from build123d import *

# Parameters (mm, degrees)
F0_W     = 90
F0_H     = 5
F1_DEPTH = 1
F0_W_2   = 5
F0_H_2   = 20
F2_DEPTH = 10
F3_W     = 90
F3_H     = 1
F4_DEPTH = 2
F5_SIZE  = 3
F6_SIZE  = 1
F7_SIZE  = 5


with BuildPart() as f1:
    # F0 (on Top) → F1 (new body)
    with BuildSketch(Plane.XY):
        with Locations((5, -7.5)):
            Rectangle(F0_W, F0_H)
    extrude(amount=F1_DEPTH)



with BuildPart() as f1b:
    # F0 (on Top) → F1, piece 2 (new body)
    with BuildSketch(Plane.XY):
        Polygon((50, 5), (50, 10), (-30, 10), (-40, 10), (-40, 5), align=None)
    extrude(amount=F1_DEPTH)


with BuildPart() as f1_1:
    add(f1.part)

    add(f1b.part)  # F2 merges F1b
    # F0 (on Top) → F2 (join)
    with BuildSketch(Plane.XY):
        Polygon((70, -10), (70, 10), (50, 10), (50, 5), (50, -5), (50, -10), align=None)
        Polygon((-45, 10), (-40, 10), (-40, 15), (-70, 15), (-70, 10), (-65, 10), align=None)
        Polygon((-40, 5), (-40, 10), (-45, 10), (-45, -10), (-40, -10), (-40, -5), align=None)
        with Locations((-67.5, 0)):
            Rectangle(F0_W_2, F0_H_2)
        Polygon((-40, -15), (-40, -10), (-45, -10), (-65, -10), (-70, -10), (-70, -15), align=None)
    extrude(amount=F2_DEPTH)

    # F3 (on face) → F4 (join)
    with BuildSketch(Plane.XY.offset(1)):
        with Locations((5, 5.5)):
            Rectangle(F3_W, F3_H)
        with Locations((5, -5.5)):
            Rectangle(F3_W, F3_H)
    extrude(amount=F4_DEPTH)

    # F5
    f5_edges = [f1_1.edges().sort_by_distance(p)[0] for p in [
        (70, -10, 5),
        (70, 10, 5),
        (50, -10, 5.5),
        (50, 10, 5.5),
    ]]
    chamfer(f5_edges, length=F5_SIZE)

    # F6
    f6_edges = [f1_1.edges().sort_by_distance(p)[0] for p in [
        (60, 10, 10),
        (51.5, 8.5, 10),
        (50, 0, 10),
        (51.5, -8.5, 10),
        (60, -10, 10),
        (68.5, -8.5, 10),
        (70, 0, 10),
        (68.5, 8.5, 10),
        (-55, 10, 10),
        (-65, 0, 10),
        (-55, -10, 10),
        (-45, 0, 10),
        (-65, 0, 0),
        (-55, -10, 0),
        (-45, 0, 0),
        (-55, 10, 0),
    ]]
    chamfer(f6_edges, length=F6_SIZE)

    # F7
    f7_edges = [f1_1.edges().sort_by_distance(p)[0] for p in [
        (-40, 15, 5),
        (-70, 15, 5),
        (-70, -15, 5),
        (-40, -15, 5),
    ]]
    chamfer(f7_edges, length=F7_SIZE)


solid = f1_1.part
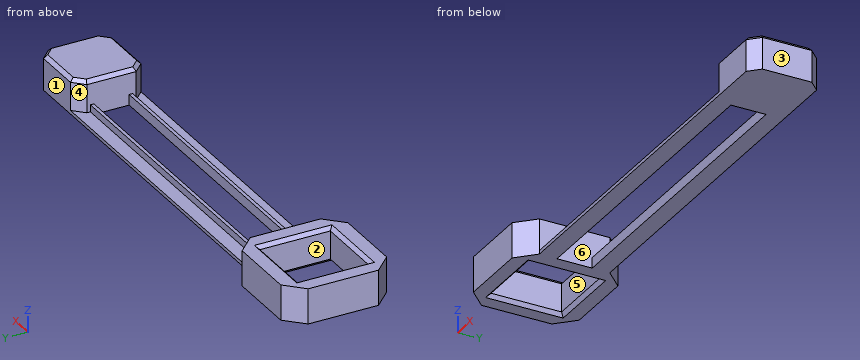
Can you work these out from the model? Positions are in its coordinate system, mm. Face numbers are marked on the shaded views. A direction names the side the tool comes from. Give positions to 0.01 mm unless a question says otherwise; leave off trailing zeros. Order: outer loops, then holes, each group sorted by start corner. A loop starts at its lowest first (then second) coordinate and runs counter-clockwise, first axis right, second up. Notation, with made-up numbers: M -34,34 L 2,34 A30 ccw 2,70 Z; hole C 85.5,35.5 d8. An arc over 180 degrees is marked long. One line per item, written item: value.
Item 1: Please list where these lines run through material, in increasing order: line 1 (X direction, y = 2, z = 8.5); line 2 (Y direction, x = -46, z = 8); line 3 (X direction, y = -9.5, z = 6).
Verdict:
line 1: -70 to -65, -45 to -40, 50 to 70
line 2: -15 to -10, 10 to 15
line 3: -70 to -65, -45 to -40, 52.5 to 67.5
Item 2: For pin 1 (0.5 mm diameter, centred on x = 19.5, y = 5.5, fed in from +Z); pin 2 (1.5 mm diameter, centred on x = 23, z = 1.5, fed in from -Y); pin 3 (5 mm diameter, centred on x = -13.5, z = 4.5, fed in from -Y), each with a flat end and sliding along its axis, tell me the tip position at first contact or that it passes through.
Verdict:
pin 1: z = 3
pin 2: y = -10
pin 3: y = -6
Item 3: If we mould it in two halves opening along X, with no side actions, what happens to the marked faces 1, 2 and 3? For each: pulls with the +X half, pulls with the -X half, needs draft (parallel to the pull), parting line crosses it, or undercut.
Verdict:
face 1: needs draft
face 2: undercut
face 3: pulls with the +X half
Item 4: If we section it at A-A on z = 5.5: Write out the boundary of the cut face in (x, y), and give its area (3 significant figures).
Verdict:
outline: M -70,-10 L -65,-15 L -45,-15 L -40,-10 L -40,10 L -45,15 L -65,15 L -70,10 Z; M 50,-7 L 53,-10 L 67,-10 L 70,-7 L 70,7 L 67,10 L 53,10 L 50,7 Z; hole M -65,-10 L -45,-10 L -45,10 L -65,10 Z
area: 832 mm2
Item 5: If we section it at C-C on x = 2.5: Write out the boundary of the cut face in (y, z).
Verdict:
outline: M -10,0 L -5,0 L -5,3 L -6,3 L -6,1 L -10,1 Z; M 5,0 L 10,0 L 10,1 L 6,1 L 6,3 L 5,3 Z
Item 6: For the marked faces 4, 5 and 6, which set-ups out of +Z, -Z, +X, -X, +Y, -Y let a thin tool reach every point of the face, with its end or its side?
Verdict:
face 4: +Z, +Y
face 5: +Z, -Z
face 6: +Z
Item 7: If we section it at B-B on x = -56.5: Write out the boundary of the cut face in (y, z), and give its area (3 significant figures).
Verdict:
outline: M -15,0 L -11,0 L -10,1 L -10,9 L -11,10 L -15,10 Z; M 10,1 L 11,0 L 15,0 L 15,10 L 11,10 L 10,9 Z
area: 98.0 mm2
